```python
from build123d import *

# Parameters (mm, degrees)
SKETCH1_R           = 13
SKETCH1_R_2         = 3
BOSS_EXTRUDE1_DEPTH = 3
SKETCH2_R           = 11.1
SKETCH2_R_2         = 1.7
BOSS_EXTRUDE2_DEPTH = 4
CHAMFER1_SIZE       = 4
CHAMFER1_SIZE_2     = 1


with BuildPart() as part:
    # Sketch1 → Boss-Extrude1 (new body)
    with BuildSketch(Plane.XY):
        with Locations((132.499999994, -1e-09)):
            Circle(SKETCH1_R)
        with Locations((132.499999994, -1e-09)):
            Circle(SKETCH1_R_2, mode=Mode.SUBTRACT)
    extrude(amount=BOSS_EXTRUDE1_DEPTH)

    # Sketch2 → Boss-Extrude2 (add)
    with BuildSketch(Plane(origin=(0, 0, 0), x_dir=(-1, 0, 0), z_dir=(0, 0, -1))):
        with Locations((-132.5, 0)):
            Circle(SKETCH2_R)
        with Locations((-132.5, 0)):
            Circle(SKETCH2_R_2, mode=Mode.SUBTRACT)
    extrude(amount=BOSS_EXTRUDE2_DEPTH)

    # Chamfer1
    # the kernel refuses this chamfer: 4, 1 mm, written as the material it takes off along each edge
    with BuildSketch(Plane(origin=(132.5, 0, -4), x_dir=(-1, 0, 0), z_dir=(0, -1, 0))) as chamfer1_piece_1_section:
        Polygon((11.1, -CHAMFER1_SIZE), (11.1 - CHAMFER1_SIZE_2, 0), (11.1, 0), align=None)
    chamfer1_piece_1 = revolve(axis=Axis((132.5, 0, -4), (0, 0, -1)), mode=Mode.PRIVATE)
    chamfer1_piece_1 = split(chamfer1_piece_1, bisect_by=Plane(origin=(132.5, 0, 0), z_dir=(0, 0, -1)), keep=Keep.TOP, mode=Mode.PRIVATE)
    add(chamfer1_piece_1, mode=Mode.SUBTRACT)


solid = part.part
```
For this review, take the finished solid that the model builds, in its own axes (mm). A direction names the side the tool comes from. Coordinates: 2 decimals unless noted, no trailing zeros. Write each loop counter-clockwise with the first axis right and the second up, starting at its lowest first coordinate (ties: lowest second). Pieces come first, ordered by that corner, then holes. Notation, with made-up numbers: (82.25, 74) -> (102.25, 74) arc R12 cw to (102.25, 88) -> close; hole circle Ø4 at (58, -12). An arc over 180 degrees is marked (long way). Put each result on its own line as item: value.
Q1. Tool access review of faces 4 (the flat face through (138, -10, 0)), 5 (the cylindrical face through (129.5, 0.1, 1.5)), 6 (the flat face through (129, 0, 3)): name each direction out of +Z, -Z, +X, -X, +Y, -Y from which nothing blocks a thin tool from reaching the whole face with its end or side.
From the geometry:
face 4: -Z
face 5: +Z
face 6: +Z, +X, -X, +Y, -Y
Q2. Take a section at C-C, the plane z = 0.5. State the section outline as (x, y) points, then the cut area to 3 significant figures.
From the geometry:
outline: circle Ø26 at (132.5, 0); hole circle Ø6 at (132.5, 0)
area: 503 mm2
Q3. Take a section at A-A, the plane y = 0. State the section outline as (x, z) points.
From the geometry:
outline: (119.5, 0) -> (121.4, 0) -> (122.4, -4) -> (130.8, -4) -> (130.8, 0) -> (129.5, 0) -> (129.5, 3) -> (119.5, 3) -> close; (134.2, -4) -> (142.6, -4) -> (143.6, 0) -> (145.5, 0) -> (145.5, 3) -> (135.5, 3) -> (135.5, 0) -> (134.2, 0) -> close
Q4. The part is to be moulded in two halves that separate along Y. For faces 1 (the cylindrical face through (144.5, -5, 1.5)), 2 (the flat face through (133, -2, -4)), 3 (the flat face through (133, -2, 0)), say which applies: +Y half, -Y half, draft (parallel to the pull), parting line (faces both ways), or undercut.
From the geometry:
face 1: parting line
face 2: draft
face 3: undercut
Q5. Take a section at D-D, the plane z = -2. State the section outline as (x, y) points.
From the geometry:
outline: circle Ø21.2 at (132.5, 0); hole circle Ø3.4 at (132.5, 0)
Q6. Clearance check with flat-ended pins moving along their axes: pin 1 Ø1.5 at (y, z) = (-7.5, 1) entering from -X; pin 2 Ø8 at (x, y) = (132.5, 0) entering from -Z; pin 3 Ø2.5 at (x, y) = (132.5, 0) entering from +Z; pin 4 Ø3 at (y, z) = (2, 0) entering from +X. State where each tip first meets the part, or that it passes through.
From the geometry:
pin 1: stops at x = 121.39
pin 2: stops at z = -4
pin 3: passes through
pin 4: stops at x = 145.49
Q7. Wall thickness on L1, parallel to Y at x = 132.5, z = 0.8; L2, parallel to X at y = 0, z = 0.9; L3, parallel to Y at x = 132.25, z = -3.25: over which ranges is each line inside the solid? List them lowest first.
From the geometry:
L1: y = -13 to -3, 3 to 13
L2: x = 119.5 to 129.5, 135.5 to 145.5
L3: y = -10.28 to -1.68, 1.68 to 10.28
Q8. Take a section at B-B, the plane x = 132.5. State the section outline as (y, z) points.
From the geometry:
outline: (-13, 0) -> (-11.1, 0) -> (-10.1, -4) -> (-1.7, -4) -> (-1.7, 0) -> (-3, 0) -> (-3, 3) -> (-13, 3) -> close; (1.7, -4) -> (10.1, -4) -> (11.1, 0) -> (13, 0) -> (13, 3) -> (3, 3) -> (3, 0) -> (1.7, 0) -> close
